Work out the finished part from the listing and answer in its coordinate system (mm). A direction names the side the tool comes from. Coordinates: 2 decimals unless noted, no trailing zeros. Loops run counter-clockwise (first coordinate to the right, second up) from the corner with the lowest first, then second, coordinate; pieces in that order, holes last. Notation, with made-up numbers: (53.5, 39.5) -> (86.5, 39.5) arc R23 cw to (86.5, 66.5) -> close; hole circle Ø11 at (51, 22). An arc over 180 degrees is marked (long way). One line per question, with ' | ' between items.
```python
from build123d import *

# Parameters (mm, degrees)
DODANIE_WYCI_GNI_CIE1_DEPTH                         = 100
M5_CLEARANCE_HOLE1_D                                = 5.5
CSK_FOR_M5_COUNTERSUNK_FLAT_HEAD_SCREW1_D           = 5.3
CSK_FOR_M5_COUNTERSUNK_FLAT_HEAD_SCREW1_CSINK_D     = 10.4
CSK_FOR_M5_COUNTERSUNK_FLAT_HEAD_SCREW1_CSINK_ANGLE = 90
CHAMFER1_SIZE                                       = 27


with BuildPart() as part:
    # Szkic1 → Dodanie-wyciągnięcie1 (new body)
    with BuildSketch(Plane.XY):
        Polygon((0, 0), (0, 30), (30, 30), (30, 0), (27, 0), (27, 27), (3, 27), (3, 0), align=None)
    extrude(amount=DODANIE_WYCI_GNI_CIE1_DEPTH)

    # M5 Clearance Hole1 (through all)
    with Locations(Plane(origin=(0, 30, 0), x_dir=(1, 0, 0), z_dir=(0, 1, 0))):
        with Locations((18, -50), (18, -15), (18, -85)):
            Hole(M5_CLEARANCE_HOLE1_D / 2)

    # CSK for M5 Countersunk Flat Head Screw1 (through all)
    with Locations(Plane(origin=(30, 0, 0), x_dir=(0, 0, -1), z_dir=(1, 0, 0))):
        with Locations((-15, 14.5), (-63, 14.5), (-39, 14.5)):
            CounterSinkHole(CSK_FOR_M5_COUNTERSUNK_FLAT_HEAD_SCREW1_D / 2, CSK_FOR_M5_COUNTERSUNK_FLAT_HEAD_SCREW1_CSINK_D / 2, counter_sink_angle=CSK_FOR_M5_COUNTERSUNK_FLAT_HEAD_SCREW1_CSINK_ANGLE)

    # Chamfer1
    chamfer1_edges = [part.edges().sort_by_distance(p)[0] for p in [
        (28.5, 0, 100),
    ]]
    chamfer(chamfer1_edges, length=CHAMFER1_SIZE)


solid = part.part
```
1) The mould has two halves that part along Y. Classify faces 1 (the face through (15, 30, 49)), 2 (the face through (16.2, 27.3, 0)), 3 (the face through (1.479, 15.296, 65.528)), 4 (the face through (15, 27, 49)): released by +Y, released by -Y, zero draft, split by the parting line, or undercut.
Check values:
face 1: released by +Y | face 2: zero draft | face 3: undercut | face 4: released by -Y
2) Find the intervals of material crossed by line 1 along Z through (x, y) = (18, 28.25); line 2 along X through (y, z) = (13.75, 48); line 3 along Y through (x, z) = (1.65, 39), in increasing order.
Check values:
line 1: z = 0 to 12.25, 17.75 to 47.25, 52.75 to 82.25, 87.75 to 100 | line 2: x = 0 to 3, 27 to 30 | line 3: y = 0 to 11.85, 17.15 to 30
3) Flat-ended cylindrical pins translate along their axes: pin 1 (7 mm diameter, centred on y = 14.5, z = 39, fed in from +X); pin 2 (8.5 mm diameter, centred on y = 14.5, z = 63, fed in from +X); pin 3 (3.5 mm diameter, centred on x = 18, z = 85, fed in from -Y); pin 4 (6 mm diameter, centred on y = 14.5, z = 63, fed in from +X). Find the tip coordinate at first contact, or state that the pin passes through.
Check values:
pin 1: stops at x = 28.3 | pin 2: stops at x = 29.05 | pin 3: passes through | pin 4: stops at x = 27.8
4) Find section C-C (z = 55.5). Write down the section's boundary in (x, y).
Check values:
outline: (0, 0) -> (3, 0) -> (3, 27) -> (27, 27) -> (27, 0) -> (30, 0) -> (30, 30) -> (0, 30) -> close
5) Find section D-D (x = 4). Write down the section's boundary in (y, z), plus the area to 3 significant figures.
Check values:
outline: (27, 0) -> (30, 0) -> (30, 100) -> (27, 100) -> close | area: 300 mm^2
6) For faces 5 (the face through (27, 13, 49)), 6 (the face through (1.48, 13.49, 17.45)), 7 (the face through (29, 14, 87)), determine the directions among +Z, -Z, +X, -X, +Y, -Y from which every point of the face is accessible in a straight line to the end or side of a thin tool.
Check values:
face 5: +Z, -Z, -Y | face 6: +X, -X | face 7: +Z, +X, -Y
7) Find section A-A (x = 18). Write down the section's boundary in (y, z), plus the area to 4 significant figures.
Check values:
outline: (27, 0) -> (30, 0) -> (30, 12.25) -> (27, 12.25) -> close; (27, 17.75) -> (30, 17.75) -> (30, 47.25) -> (27, 47.25) -> close; (27, 52.75) -> (30, 52.75) -> (30, 82.25) -> (27, 82.25) -> close; (27, 87.75) -> (30, 87.75) -> (30, 100) -> (27, 100) -> close | area: 250.5 mm^2
8) Find section B-B (z = 39). Write down the section's boundary in (x, y), plus the area to 3 significant figures.
Check values:
outline: (0, 0) -> (3, 0) -> (3, 11.85) -> (0, 11.85) -> close; (0, 17.15) -> (3, 17.15) -> (3, 27) -> (27, 27) -> (27, 17.15) -> (27.45, 17.15) -> (30, 19.7) -> (30, 30) -> (0, 30) -> close; (27, 0) -> (30, 0) -> (30, 9.3) -> (27.45, 11.85) -> (27, 11.85) -> close | area: 214 mm^2
